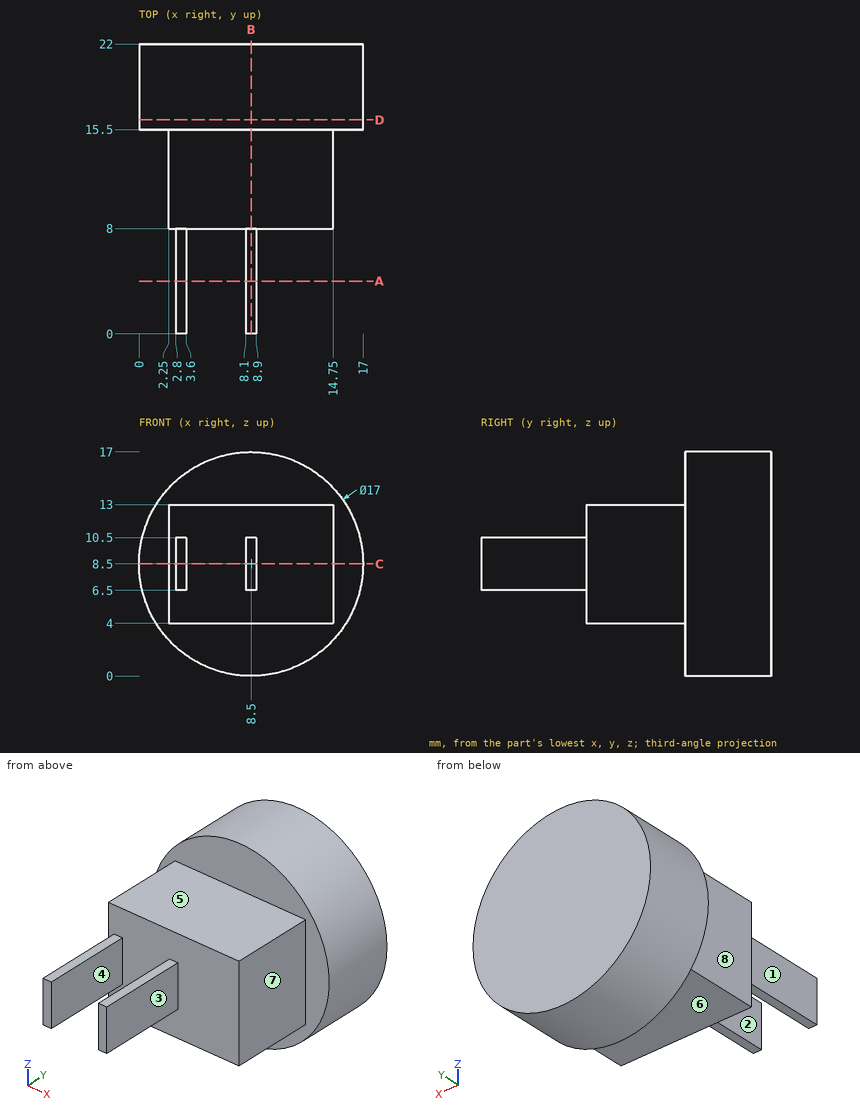
Study the drawing (mm; zero at the part's minimum x, y, z) and answer. A direction names the side the tool comes from. Give positions to 0.01 mm unless a question says otherwise; leave off trailing zeros. Order: outer loops, then holes, each group sorted by start corner. A loop starts at its lowest first (then second) coordinate and runs counter-clockwise, first axis right, second up. Notation, with made-up numbers: (-0.75, 0.5) - (33.25, 0.5) arc R23 cw to (33.25, 38.5) - close; hole circle Ø8 at (-16.75, 66). An arc over 180 degrees is marked (long way). Use one line per item in the form item = value. Start each with the question number.
(1) For the marked faces 5, 6, 7 and 8, determine the directions among +Z, -Z, +X, -X, +Y, -Y from which every point of the face is accessible in a straight line to the end or side of a thin tool.
(2) Flat-ended cylindrical pins translate along their axes: pin 1 Ø7 at (x, z) = (7, 8) entering from -Y; pin 2 Ø3 at (y, z) = (4.5, 8.5) entering from -X; pin 3 Ø4 at (y, z) = (19, 4.5) entering from -X; pin 4 Ø0.6 at (x, y) = (8.5, 5.5) entering from +Z. Find the tip coordinate at first contact, or state that the pin passes through.
(3) Consider line 1 (X direction, y = 1.75, z = 8.5); line 2 (Y direction, x = 16, z = 8.5); line 3 (Z direction, x = 3.75, y = 14). Determine where each line is inside the solid, lowest interval first. Write a range as from..to.
(4) A cutting plane is placed at C-C, the plane z = 8.5. Write down the section's boundary in (x, y), then the cut area to 3 significant figures.
(5) A cutting plane is placed at B-B, the plane x = 8.5. Write down the section's boundary in (y, z), then the cut area to 3 significant figures.
(6) A cutting plane is placed at D-D, the plane y = 16.25. Write down the section's boundary in (x, z).
(7) A cutting plane is placed at A-A, the plane y = 4. Write down the section's boundary in (x, z), then the cut area to 3 significant figures.
(8) The mould has two halves that part along X. Classify the marked faces 1, 2, 3 and 4: released by +X, released by -X, zero draft, split by the parting line, or undercut.
Ans:
q1.face_5 = +Z, +X, -X, -Y
q1.face_6 = -Z, +X, -X, -Y
q1.face_7 = +Z, -Z, +X, -Y
q1.face_8 = +Z, -Z, -X, -Y
q2.pin_1 = 0
q2.pin_2 = 2.8
q2.pin_3 = 0.24
q2.pin_4 = 10.5
q3.line_1 = 2.8..3.6, 8.1..8.9
q3.line_2 = 15.5..22
q3.line_3 = 4..13
q4.outline = (0, 15.5) - (2.25, 15.5) - (2.25, 8) - (2.8, 8) - (2.8, 0) - (3.6, 0) - (3.6, 8) - (8.1, 8) - (8.1, 0) - (8.9, 0) - (8.9, 8) - (14.75, 8) - (14.75, 15.5) - (17, 15.5) - (17, 22) - (0, 22) - close
q4.area = 217 mm^2
q5.outline = (0, 6.5) - (8, 6.5) - (8, 4) - (15.5, 4) - (15.5, 0) - (22, 0) - (22, 17) - (15.5, 17) - (15.5, 13) - (8, 13) - (8, 10.5) - (0, 10.5) - close
q5.area = 210 mm^2
q6.outline = circle Ø17 at (8.5, 8.5)
q7.outline = (2.8, 6.5) - (3.6, 6.5) - (3.6, 10.5) - (2.8, 10.5) - close; (8.1, 6.5) - (8.9, 6.5) - (8.9, 10.5) - (8.1, 10.5) - close
q7.area = 6.40 mm^2
q8.face_1 = released by -X
q8.face_2 = undercut
q8.face_3 = released by +X
q8.face_4 = undercut
